from build123d import *

# Parameters (mm, degrees)
SKETCH_2_R      = 1.5
EXTRUDE_1_DEPTH = 1.5
SKETCH_3_W      = 22.5
SKETCH_3_H      = 10
SKETCH_3_W_2    = 12
SKETCH_3_W_3    = 10
SKETCH_3_H_2    = 12
SKETCH_3_H_3    = 22.5
SKETCH_3_W_4    = 18
EXTRUDE_2_DEPTH = 5
SKETCH_4_W      = 6
SKETCH_4_H      = 20
EXTRUDE_3_DEPTH = 15
FILLET_1_R      = 10
SKETCH_6_W      = 13.5
SKETCH_6_H      = 20
SKETCH_6_W_2    = 13
SKETCH_6_H_2    = 25
EXTRUDE_5_DEPTH = 3


with BuildPart() as part:
    # 草图2 → 凸台-拉伸1 (new body)
    # profile 1 of 3: a face of its own
    with BuildSketch(Plane(origin=(0, 0, 0), x_dir=(1, 0, 0), z_dir=(0, 1, 0))):
        with BuildLine():
            Line((250.604175692, 167.040097328), (237.354175692, 167.040097328))
            Line((237.354175692, 167.040097328), (229.354175692, 159.040097328))
            Line((229.354175692, 159.040097328), (229.354175692, 157.622673023))
            ThreePointArc((229.354175692, 157.622673023), (231.537475825, 155.778710115), (232.354175692, 153.040097328))
            ThreePointArc((232.354175692, 153.040097328), (231.537475825, 150.30148454), (229.354175692, 148.457521633))
            Line((229.354175692, 148.457521633), (229.354175692, 144.040097328))
            Line((229.354175692, 144.040097328), (232.354175692, 144.040097328))
            Line((232.354175692, 144.040097328), (232.354175692, 108.040097328))
            Line((232.354175692, 108.040097328), (229.354175692, 108.040097328))
            Line((229.354175692, 108.040097328), (229.354175692, 104.622673023))
            ThreePointArc((229.354175692, 104.622673023), (231.537475825, 102.778710115), (232.354175692, 100.040097328))
            ThreePointArc((232.354175692, 100.040097328), (231.537475825, 97.30148454), (229.354175692, 95.457521633))
            Line((229.354175692, 95.457521633), (229.354175692, 89.040097328))
            Line((229.354175692, 89.040097328), (248.966003356, 62.564129981))
            ThreePointArc((248.966003356, 62.564129981), (249.273338447, 62.30138118), (249.581919942, 62.040097328))
            Line((249.581919942, 62.040097328), (316.354175692, 62.040097328))
            Line((316.354175692, 62.040097328), (316.354175692, 72.040097328))
            Line((316.354175692, 72.040097328), (334.354175692, 72.040097328))
            Line((334.354175692, 72.040097328), (334.354175692, 62.040097328))
            Line((334.354175692, 62.040097328), (359.126431443, 62.040097328))
            ThreePointArc((359.126431443, 62.040097328), (359.435012937, 62.30138118), (359.742348028, 62.564129981))
            Line((359.742348028, 62.564129981), (379.354175692, 89.040097328))
            Line((379.354175692, 89.040097328), (379.354175692, 95.457521633))
            ThreePointArc((379.354175692, 95.457521633), (376.354175692, 100.040097328), (379.354175692, 104.622673023))
            Line((379.354175692, 104.622673023), (379.354175692, 108.040097328))
            Line((379.354175692, 108.040097328), (376.354175692, 108.040097328))
            Line((376.354175692, 108.040097328), (376.354175692, 144.040097328))
            Line((376.354175692, 144.040097328), (379.354175692, 144.040097328))
            Line((379.354175692, 144.040097328), (379.354175692, 148.457521633))
            ThreePointArc((379.354175692, 148.457521633), (376.354175692, 153.040097328), (379.354175692, 157.622673023))
            Line((379.354175692, 157.622673023), (379.354175692, 159.040097328))
            Line((379.354175692, 159.040097328), (371.354175692, 167.040097328))
            Line((371.354175692, 167.040097328), (358.104175692, 167.040097328))
            Line((358.104175692, 167.040097328), (358.104175692, 164.040097328))
            Line((358.104175692, 164.040097328), (322.104175692, 164.040097328))
            Line((322.104175692, 164.040097328), (322.104175692, 167.040097328))
            Line((322.104175692, 167.040097328), (315.604175692, 167.040097328))
            Line((315.604175692, 167.040097328), (315.604175692, 164.040097328))
            Line((315.604175692, 164.040097328), (293.104175692, 164.040097328))
            Line((293.104175692, 164.040097328), (293.104175692, 167.040097328))
            Line((293.104175692, 167.040097328), (286.604175692, 167.040097328))
            Line((286.604175692, 167.040097328), (286.604175692, 164.040097328))
            Line((286.604175692, 164.040097328), (250.604175692, 164.040097328))
            Line((250.604175692, 164.040097328), (250.604175692, 167.040097328))
        make_face()
        with Locations(Location((234.354175692, 105.052003777, 0), (0, 0, 270))):
            Circle(SKETCH_2_R, mode=Mode.SUBTRACT)
        with Locations(Location((374.354175692, 105.052003777, 0), (0, 0, 270))):
            Circle(SKETCH_2_R, mode=Mode.SUBTRACT)
        with Locations(Location((233.354175692, 147.040097328, 0), (0, 0, 270))):
            Circle(SKETCH_2_R, mode=Mode.SUBTRACT)
        with Locations(Location((375.354175692, 147.040097328, 0), (0, 0, 270))):
            Circle(SKETCH_2_R, mode=Mode.SUBTRACT)
    # profile 2 of 3: a face of its own
    with BuildSketch(Plane(origin=(0, 0, 0), x_dir=(1, 0, 0), z_dir=(0, 1, 0))):
        with BuildLine():
            ThreePointArc((249.581919942, 62.040097328), (249.273338447, 62.30138118), (248.966003356, 62.564129981))
            Line((248.966003356, 62.564129981), (249.354175692, 62.040097328))
            Line((249.354175692, 62.040097328), (249.581919942, 62.040097328))
        make_face()
    # profile 3 of 3: a face of its own
    with BuildSketch(Plane(origin=(0, 0, 0), x_dir=(1, 0, 0), z_dir=(0, 1, 0))):
        with BuildLine():
            ThreePointArc((359.742348028, 62.564129981), (359.435012937, 62.30138118), (359.126431443, 62.040097328))
            Line((359.126431443, 62.040097328), (359.354175692, 62.040097328))
            Line((359.354175692, 62.040097328), (359.742348028, 62.564129981))
        make_face()
    extrude(amount=EXTRUDE_1_DEPTH)

    # 草图3 → 凸台-拉伸2 (add)
    with BuildSketch(Plane(origin=(0, 1.5, 0), x_dir=(1, 0, 0), z_dir=(0, 1, 0))):
        with Locations((261.854175692, 156.040097328)):
            Rectangle(SKETCH_3_W, SKETCH_3_H)
        with Locations((280.604175692, 156.040097328)):
            Rectangle(SKETCH_3_W_2, SKETCH_3_H)
        with Locations((304.354175692, 156.040097328)):
            Rectangle(SKETCH_3_W, SKETCH_3_H)
        with Locations((328.104175692, 156.040097328)):
            Rectangle(SKETCH_3_W_2, SKETCH_3_H)
        with Locations((346.854175692, 156.040097328)):
            Rectangle(SKETCH_3_W, SKETCH_3_H)
        with Locations((368.354175692, 138.040097328)):
            Rectangle(SKETCH_3_W_3, SKETCH_3_H_2)
        with Locations((368.354175692, 119.290097328)):
            Rectangle(SKETCH_3_W_3, SKETCH_3_H_3)
        with Locations((240.354175692, 138.040097328)):
            Rectangle(SKETCH_3_W_3, SKETCH_3_H_2)
        with Locations((240.354175692, 119.290097328)):
            Rectangle(SKETCH_3_W_3, SKETCH_3_H_3)
        Polygon((232.647068911, 158.090349859), (238.30392316, 163.747204109), (245.374990972, 156.676136297), (239.718136723, 151.019282048), align=None)
        Polygon((369.697321443, 164.45431089), (376.768389254, 157.383243078), (369.697321443, 150.312175266), (362.626253631, 157.383243078), align=None)
        with Locations((325.354175692, 77.040097328)):
            Rectangle(SKETCH_3_W_4, SKETCH_3_H)
    extrude(amount=EXTRUDE_2_DEPTH)

    # 草图4 → 凸台-拉伸3 (add)
    with BuildSketch(Plane(origin=(0, 1.5, 0), x_dir=(1, 0, 0), z_dir=(0, 1, 0))):
        with Locations((346.354175692, 117.040097328)):
            Rectangle(SKETCH_4_W, SKETCH_4_H)
    extrude(amount=EXTRUDE_3_DEPTH)

    # 圆角1
    # the kernel refuses this fillet: 10 mm, written as the material it takes off along each edge
    with BuildSketch(Plane(origin=(229.354175692, -8.403282896, -159.040097328), x_dir=(0.7071067811865475, 0, -0.7071067811865475), z_dir=(0, 1, 0))) as fillet_1_piece_1:
        with BuildLine():
            CenterArc((3.361313158, -10), FILLET_1_R, 90, 25.871759313)
            Line((-1.002270338, -1.002270338), (-1.089542008, -0.822315745))
            ThreePointArc((-1.089542008, -0.822315745), (-0.642556525, -0.359713813), (-0.141421356, 0.141421356))
            Line((-0.141421356, 0.141421356), (0, 0.2))
            Line((0, 0.2), (3.361313158, 0.2))
            Line((3.361313158, 0.2), (3.361313158, 0))
        make_face()
    extrude(amount=18.306565791, mode=Mode.SUBTRACT)
    with BuildSketch(Plane(origin=(237.354175692, -10.355339059, -167.040097328), x_dir=(1, 0, 0), z_dir=(0, 1, 0)), Plane(origin=(371.354175692, -10.355339059, -167.040097328), x_dir=(0.707106781186544, 0, 0.7071067811865509), z_dir=(0, 1, 0))) as fillet_1_piece_2:
        with BuildLine():
            CenterArc((FILLET_1_R * 0.414213562373, -FILLET_1_R), FILLET_1_R, 90, 45)
            Line((-FILLET_1_R * 0.292893218813, -FILLET_1_R * 0.292893218813), (-FILLET_1_R * 0.307035354437, -FILLET_1_R * 0.27875108319))
            Line((-FILLET_1_R * 0.307035354437, -FILLET_1_R * 0.27875108319), (-FILLET_1_R * 0.00828427124746, FILLET_1_R * 0.02))
            Line((-FILLET_1_R * 0.00828427124746, FILLET_1_R * 0.02), (FILLET_1_R * 0.414213562373, FILLET_1_R * 0.02))
            Line((FILLET_1_R * 0.414213562373, FILLET_1_R * 0.02), (FILLET_1_R * 0.414213562373, 0))
        make_face()
    extrude(amount=22.210678119, mode=Mode.SUBTRACT)
    with BuildSketch(Plane(origin=(379.354175692, -8.403282896, -159.040097328), x_dir=(0, 0, 1), z_dir=(0, 1, 0))) as fillet_1_piece_3:
        with BuildLine():
            CenterArc((4.694260484, -9.44787514), FILLET_1_R, 109.128240687, 25.871759313)
            Line((-2.376807328, -2.376807328), (-2.518228684, -2.235385972))
            Line((-2.518228684, -2.235385972), (-0.141421356, 0.141421356))
            Line((-0.141421356, 0.141421356), (0, 0.2))
            ThreePointArc((0, 0.2), (0.708712153, 0.2), (1.351887581, 0.188957503))
            Line((1.351887581, 0.188957503), (1.417424305, 0))
        make_face()
    extrude(amount=18.306565791, mode=Mode.SUBTRACT)
    with BuildSketch(Plane(origin=(379.354175692, -8.250744041, -89.040097328), x_dir=(0, 0, -1), z_dir=(0, 1, 0))) as fillet_1_piece_4:
        with BuildLine():
            CenterArc((FILLET_1_R * 0.330029761641, FILLET_1_R), FILLET_1_R, 233.471144633, 36.528855367)
            Line((-FILLET_1_R * 0.265197788985, FILLET_1_R * 0.196442806655), (-FILLET_1_R * 0.277102339997, FILLET_1_R * 0.180371662788))
            Line((-FILLET_1_R * 0.277102339997, FILLET_1_R * 0.180371662788), (-FILLET_1_R * 0.00660059523282, -FILLET_1_R * 0.02))
            Line((-FILLET_1_R * 0.00660059523282, -FILLET_1_R * 0.02), (FILLET_1_R * 0.330029761641, -FILLET_1_R * 0.02))
            Line((FILLET_1_R * 0.330029761641, -FILLET_1_R * 0.02), (FILLET_1_R * 0.330029761641, 0))
        make_face()
    extrude(amount=18.001488082, mode=Mode.SUBTRACT)
    with BuildSketch(Plane(origin=(359.354175692, -12.593143734, -62.040097328), x_dir=(0.5952275506257363, 0, -0.8035571933447467), z_dir=(0, 1, 0))) as fillet_1_piece_5:
        with BuildLine():
            CenterArc((FILLET_1_R * 0.503725749364, FILLET_1_R), FILLET_1_R, 216.528855367, 53.471144633)
            Line((-FILLET_1_R * 0.299831443981, FILLET_1_R * 0.404772449374), (-FILLET_1_R * 0.315902587848, FILLET_1_R * 0.392867898362))
            Line((-FILLET_1_R * 0.315902587848, FILLET_1_R * 0.392867898362), (-FILLET_1_R * 0.0100745149873, -FILLET_1_R * 0.02))
            Line((-FILLET_1_R * 0.0100745149873, -FILLET_1_R * 0.02), (FILLET_1_R * 0.503725749364, -FILLET_1_R * 0.02))
            Line((FILLET_1_R * 0.503725749364, -FILLET_1_R * 0.02), (FILLET_1_R * 0.503725749364, 0))
        make_face()
    extrude(amount=26.686287468, mode=Mode.SUBTRACT)
    with BuildSketch(Plane(origin=(249.354175692, -12.593143734, -62.040097328), x_dir=(-0.5952275506257363, 0, -0.8035571933447467), z_dir=(0, 1, 0))) as fillet_1_piece_6:
        with BuildLine():
            CenterArc((FILLET_1_R * 0.503725749364, -FILLET_1_R), FILLET_1_R, 90, 53.471144633)
            Line((-FILLET_1_R * 0.299831443981, -FILLET_1_R * 0.404772449374), (-FILLET_1_R * 0.315902587848, -FILLET_1_R * 0.392867898362))
            Line((-FILLET_1_R * 0.315902587848, -FILLET_1_R * 0.392867898362), (-FILLET_1_R * 0.0100745149873, FILLET_1_R * 0.02))
            Line((-FILLET_1_R * 0.0100745149873, FILLET_1_R * 0.02), (FILLET_1_R * 0.503725749364, FILLET_1_R * 0.02))
            Line((FILLET_1_R * 0.503725749364, FILLET_1_R * 0.02), (FILLET_1_R * 0.503725749364, 0))
        make_face()
    extrude(amount=26.686287468, mode=Mode.SUBTRACT)
    with BuildSketch(Plane(origin=(229.354175692, -8.250744041, -89.040097328), x_dir=(0, 0, -1), z_dir=(0, 1, 0))) as fillet_1_piece_7:
        with BuildLine():
            CenterArc((FILLET_1_R * 0.330029761641, -FILLET_1_R), FILLET_1_R, 90, 36.528855367)
            Line((-FILLET_1_R * 0.265197788985, -FILLET_1_R * 0.196442806655), (-FILLET_1_R * 0.277102339997, -FILLET_1_R * 0.180371662788))
            Line((-FILLET_1_R * 0.277102339997, -FILLET_1_R * 0.180371662788), (-FILLET_1_R * 0.00660059523282, FILLET_1_R * 0.02))
            Line((-FILLET_1_R * 0.00660059523282, FILLET_1_R * 0.02), (FILLET_1_R * 0.330029761641, FILLET_1_R * 0.02))
            Line((FILLET_1_R * 0.330029761641, FILLET_1_R * 0.02), (FILLET_1_R * 0.330029761641, 0))
        make_face()
    extrude(amount=18.001488082, mode=Mode.SUBTRACT)

    # 草图6 → 凸台-拉伸5 (add)
    with BuildSketch(Plane(origin=(0, 1.5, 0), x_dir=(1, 0, 0), z_dir=(0, 1, 0))):
        with Locations((262.104175692, 72.040097328)):
            Rectangle(SKETCH_6_W, SKETCH_6_H)
        with Locations((346.854175692, 74.540097328)):
            Rectangle(SKETCH_6_W_2, SKETCH_6_H_2)
    extrude(amount=EXTRUDE_5_DEPTH)


solid = part.part
Source: CAD feature listing. Evaluate the final solid. Frame: model axes, mm. A direction names the side the tool comes from. Give positions to 0.01 mm unless a question says otherwise; leave off trailing zeros. Order: outer loops, then holes, each group sorted by start corner. A loop starts at its lowest first (then second) coordinate and runs counter-clockwise, first axis right, second up. Notation, with made-up numbers: (9, -2.75) -> (55, -2.75) arc R17 cw to (55, 12.25) -> close; hole circle Ø5 at (24, 80). An arc over 180 degrees is marked (long way). Use a Markdown table: item, result.
1) Section query C-C, the plane y = 11.5. Return the cut outline in (x, z), then the cut area to 3 significant figures.
Answer list:
| item | result |
|---|---|
| outline | (343.35, -127.04) -> (349.35, -127.04) -> (349.35, -107.04) -> (343.35, -107.04) -> close |
| area | 120 mm² |
2) Section query D-D, the plane z = -122. Return the cut outline in (x, y).
Answer list:
| item | result |
|---|---|
| outline | (232.35, 0) -> (376.35, 0) -> (376.35, 1.5) -> (373.35, 1.5) -> (373.35, 6.5) -> (363.35, 6.5) -> (363.35, 1.5) -> (349.35, 1.5) -> (349.35, 16.5) -> (343.35, 16.5) -> (343.35, 1.5) -> (245.35, 1.5) -> (245.35, 6.5) -> (235.35, 6.5) -> (235.35, 1.5) -> (232.35, 1.5) -> close |
3) Reachability of faces 4 (the flat face through (235.354, 4, -119)), 5 (the flat face through (340.354, 3, -74)), 6 (the flat face through (334.354, 4, -77)), 7 (the flat face through (325, 4, -82.04)) from +Z, -Z, +X, -X, +Y, -Y: full face, straight path, thin tool, end or side. Return the list, or none.
Answer list:
| item | result |
|---|---|
| face 4 | +Z, -X, +Y |
| face 5 | +Z, +Y |
| face 6 | +Z, -Z, +Y |
| face 7 | -X, +Y |
4) Mould query, pull axis X, two halves, no side actions, for faces 1 (the flat face through (303, 0, -115)), 2 (the cylindrical face through (235.368, 0.74, -106.158)), 3 (the flat face through (373.282, 3.965, -153.897)). Classes: +X half, -X half, draft (parallel to the pull), parting line (faces both ways), or undercut.
Answer list:
| item | result |
|---|---|
| face 1 | draft |
| face 2 | undercut |
| face 3 | +X half |
5) Section query A-A, the plane x = 324. Return the cut outline in (y, z), then the cut area to 3 significant figures.
Answer list:
| item | result |
|---|---|
| outline | (0, -164.04) -> (1.5, -164.04) -> (1.5, -161.04) -> (6.5, -161.04) -> (6.5, -151.04) -> (1.5, -151.04) -> (1.5, -82.04) -> (6.5, -82.04) -> (6.5, -72.04) -> (0, -72.04) -> close |
| area | 238 mm² |
6) Section query B-B, the plane z = -68.5. Return the cut outline in (x, y).
Answer list:
| item | result |
|---|---|
| outline | (244.57, 0) -> (316.35, 0) -> (316.35, 1.5) -> (268.85, 1.5) -> (268.85, 4.5) -> (255.35, 4.5) -> (255.35, 1.5) -> (244.57, 1.5) -> close; (334.35, 0) -> (364.14, 0) -> (364.14, 1.5) -> (353.35, 1.5) -> (353.35, 4.5) -> (340.35, 4.5) -> (340.35, 1.5) -> (334.35, 1.5) -> close |
7) Contact query for flat-ended pins moving along their axis: P1, Ø4, axis at y = 4, z = -157.5, coming from the -X side; P2, Ø5.5, axis at y = 4.5, z = -76.5, coming from the +X side; P3, Ø4, axis at x = 309, y = 5, coming from the -Z side; P4, Ø2, axis at x = 291, y = 7.5, coming from the +Z side. Output: stop coordinate, or through.
Answer list:
| item | result |
|---|---|
| P1 | x = 232.65 |
| P2 | x = 353.35 |
| P3 | z = -161.04 |
| P4 | through |
8) Ray query, line 1 along X through (y, z) = (5, -130.5); line 2 along Z through (x, y) = (262, 4.25); line 3 along Z through (x, y) = (319, 3.25). Return the intervals inside material, ascending. Write a range as [from, to].
Answer list:
| item | result |
|---|---|
| line 1 | [235.35, 245.35], [363.35, 373.35] |
| line 2 | [-161.04, -151.04], [-82.04, -62.04] |
| line 3 | [-82.04, -72.04] |
